Geometry check sheet. Reference: drawing and pictorial views, mm from the part's lowest x, y, z. Round coordinates to 2 decimals unless told otherwise and drop trailing zeros. Order: outer loops, then holes, each group sorted by start corner. A loop starts at its lowest first (then second) coordinate and runs counter-clockwise, first axis right, second up. Notation, with made-up numbers: (-20.5, -17.75) -> (17.5, -17.75) arc R38 cw to (17.5, 21.25) -> close; hole circle Ø8 at (-0.5, -0.75). An arc over 180 degrees is marked (long way). Return JSON: item names as keys, results as strings. Group by question number.
1) Scan lines: L1, parallel to X at y = 2, z = 6; L2, parallel to X at y = 1.15, z = 117 (1 decimal); L3, parallel to X at y = 3.75, z = 64 (1 decimal). Record each from-to range of solid material in increasing order.
2) Section check D-D on x = 100. Enter the section's corners in (y, z).
3) Section check B-B on z = 61.5. Enter the section's corners in (x, y).
4) Depth check by flat-ended pin: pin 1 (1.5 mm diameter, centred on x = 42, z = 59.5, fed in from -Y); pin 2 (4 mm diameter, centred on x = 6, z = 6, fed in from +Y); pin 3 (5.5 mm diameter, centred on x = 6, z = 117, fed in from +Y); pin 4 (2 mm diameter, centred on x = 6, z = 61.5, fed in from -Y). Enter the tip coordinate at first touch or a pass-through.
5) Section check A-A on z = 6. Enter the section's corners in (x, y).
6) Section check C-C on x = 53. Enter the section's corners in (y, z), plus the area to 3 significant figures.
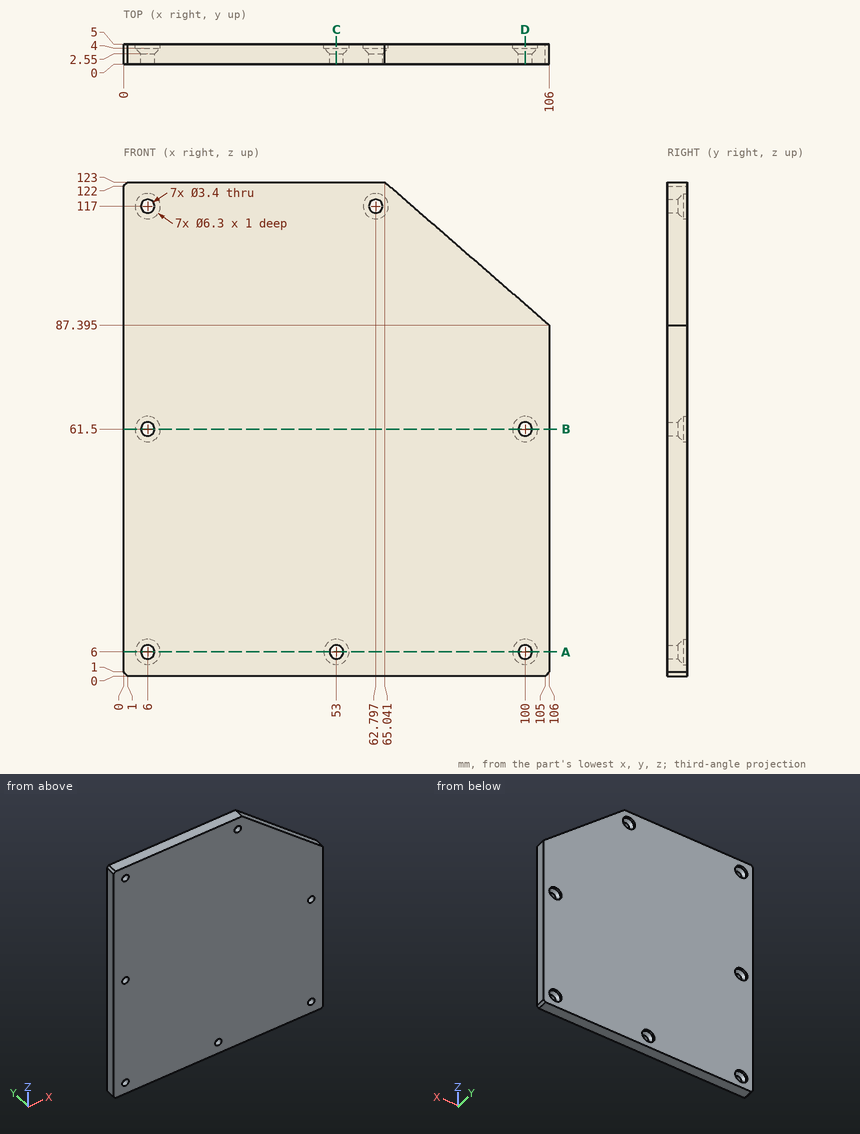
Check result:
{
 "1": {"L1": "0 to 4.3, 7.7 to 51.3, 54.7 to 98.3, 101.7 to 106", "L2": "0 to 4.3, 7.7 to 61.1, 64.5 to 71.9", "L3": "0 to 4.5, 7.5 to 98.5, 101.5 to 106"},
 "2": {"outline": "(0, 0) -> (5, 0) -> (5, 2.85) -> (4, 2.85) -> (2.55, 4.3) -> (0, 4.3) -> close; (0, 7.7) -> (2.55, 7.7) -> (4, 9.15) -> (5, 9.15) -> (5, 58.35) -> (4, 58.35) -> (2.55, 59.8) -> (0, 59.8) -> close; (0, 63.2) -> (2.55, 63.2) -> (4, 64.65) -> (5, 64.65) -> (5, 92.61) -> (0, 92.61) -> close"},
 "3": {"outline": "(0, 0) -> (4.3, 0) -> (4.3, 2.55) -> (2.85, 4) -> (2.85, 5) -> (0, 5) -> close; (7.7, 0) -> (98.3, 0) -> (98.3, 2.55) -> (96.85, 4) -> (96.85, 5) -> (9.15, 5) -> (9.15, 4) -> (7.7, 2.55) -> close; (101.7, 0) -> (106, 0) -> (106, 5) -> (103.15, 5) -> (103.15, 4) -> (101.7, 2.55) -> close"},
 "4": {"pin 1": "y = 0", "pin 2": "y = 2.85", "pin 3": "y = 3.6", "pin 4": "through"},
 "5": {"outline": "(0, 0) -> (4.3, 0) -> (4.3, 2.55) -> (2.85, 4) -> (2.85, 5) -> (0, 5) -> close; (7.7, 0) -> (51.3, 0) -> (51.3, 2.55) -> (49.85, 4) -> (49.85, 5) -> (9.15, 5) -> (9.15, 4) -> (7.7, 2.55) -> close; (54.7, 0) -> (98.3, 0) -> (98.3, 2.55) -> (96.85, 4) -> (96.85, 5) -> (56.15, 5) -> (56.15, 4) -> (54.7, 2.55) -> close; (101.7, 0) -> (106, 0) -> (106, 5) -> (103.15, 5) -> (103.15, 4) -> (101.7, 2.55) -> close"},
 "6": {"outline": "(0, 0) -> (5, 0) -> (5, 2.85) -> (4, 2.85) -> (2.55, 4.3) -> (0, 4.3) -> close; (0, 7.7) -> (2.55, 7.7) -> (4, 9.15) -> (5, 9.15) -> (5, 123) -> (0, 123) -> close", "area": "593 mm^2"}
}
